```python
from build123d import *

# Parameters (mm, degrees)
F0_W     = 91
F0_H     = 33
F0_W_2   = 33
F0_H_2   = 13
F0_H_3   = 51
F1_DEPTH = 2
F2_D     = 4
F3_D     = 10


with BuildPart() as f1:
    # F0 (on Top) → F1 (new body)
    with BuildSketch(Plane.XY):
        Polygon((45.5, 9), (45.5, 25.5), (-45.5, 25.5), (-45.5, -25.5), (45.5, -25.5), (45.5, -9), (40.5, -9), (40.5, 9), align=None)
        Polygon((78.5, 25.5), (45.5, 25.5), (45.5, 9), (45.5, -9), (45.5, -25.5), (78.5, -25.5), align=None)
        with Locations((0, 42)):
            Rectangle(F0_W, F0_H)
        with Locations((-26, 34)):
            Rectangle(F0_W_2, F0_H_2, mode=Mode.SUBTRACT)
        with Locations((-62, 0)):
            Rectangle(F0_W_2, F0_H_3)
        with Locations((0, -42)):
            Rectangle(F0_W, F0_H)
        Polygon((-24.5, -40.5), (-42.5, -40.5), (-42.5, -27.5), (-24.5, -27.5), (-24.5, -30.5), (-14.5, -30.5), (-14.5, -35.5), (-24.5, -35.5), align=None, mode=Mode.SUBTRACT)
    extrude(amount=F1_DEPTH)

    # F2 (through all)
    with Locations(Plane(origin=(0, 0, 0), x_dir=(1, 0, 0), z_dir=(0, 0, -1))):
        with Locations((-20, 53.5), (20, -53.5)):
            Hole(F2_D / 2)

    # F3 (through all)
    with Locations(Plane(origin=(0, 0, 0), x_dir=(1, 0, 0), z_dir=(0, 0, -1))):
        with Locations((0, -7), (0, 7)):
            Hole(F3_D / 2)


solid = f1.part
```
Here's how the part is built. I have some questions about the finished solid (model axes, mm). Round coordinates to 2 decimals unless told otherwise and drop trailing zeros. Order: outer loops, then holes, each group sorted by start corner. A loop starts at its lowest first (then second) coordinate and runs counter-clockwise, first axis right, second up. Notation, with made-up numbers: M -29.75,20 L 17.25,20 A23 cw 17.25,56 Z; hole C 54,34.25 d1. An arc over 180 degrees is marked long. Use CSV: the item, a comma, the result in double quotes.
1) I'm going to push flat-ended pins straight in: P1, Ø1, axis at y = -32, z = 1, coming from the -X side; P2, Ø3, axis at x = -20, y = -53.5, coming from the +Z side; P3, Ø1, axis at y = -37, z = 1, coming from the +X side. Where does each tip first touch, or does it pass through?
Taken from the geometry:
P1,"x = -45.5"
P2,"through"
P3,"x = 45.5"
2) I want a section at B-B (x = 0). List the corners of the cut face in (y, z) for me, then the cut area to 3 significant figures.
Taken from the geometry:
outline,"M -58.5,0 L -12,0 L -12,2 L -58.5,2 Z; M -2,0 L 2,0 L 2,2 L -2,2 Z; M 12,0 L 58.5,0 L 58.5,2 L 12,2 Z"
area,"194 mm^2"
3) I want a section at D-D (y = -53.5). List the corners of the cut face in (x, z) for me.
Taken from the geometry:
outline,"M -45.5,0 L -22,0 L -22,2 L -45.5,2 Z; M -18,0 L 45.5,0 L 45.5,2 L -18,2 Z"
4) I want a section at C-C (z = 0.7). Count the separate pieces of the cut face and the enclosed holes in it, then the cut area to 3 significant figures.
Taken from the geometry:
separate pieces,"1"
enclosed holes,"7"
area,"13,000 mm^2"
5) I want a section at A-A (y = -7). List the corners of the cut face in (x, z) for me, then the cut area to 3 significant figures.
Taken from the geometry:
outline,"M -78.5,0 L -5,0 L -5,2 L -78.5,2 Z; M 5,0 L 40.5,0 L 40.5,2 L 5,2 Z; M 45.5,0 L 78.5,0 L 78.5,2 L 45.5,2 Z"
area,"284 mm^2"
6) If we mould it in two halves opening along X, with no side actions, what happens to faces 1 (the flat face through (-1, 1, 2)), 2 (the cylindrical face through (-3, 3, 1))? For each: pulls with the +X half, pulls with the -X half, needs draft (parallel to the pull), parting line crosses it, or undercut.
Taken from the geometry:
face 1,"needs draft"
face 2,"undercut"
7) I need wall thicknesses on line 1 along Y through (x, z) = (-29, 0.85); line 2 along Y through (x, z) = (0, 1.35); line 3 along Y through (x, z) = (-20, 1). Which ranges of each line are inside material? Lowest first, please. Write a range as [from, to].
Taken from the geometry:
line 1,"[-58.5, -40.5], [-27.5, 27.5], [40.5, 58.5]"
line 2,"[-58.5, -12], [-2, 2], [12, 58.5]"
line 3,"[-58.5, -55.5], [-51.5, -35.5], [-30.5, 27.5], [40.5, 58.5]"
